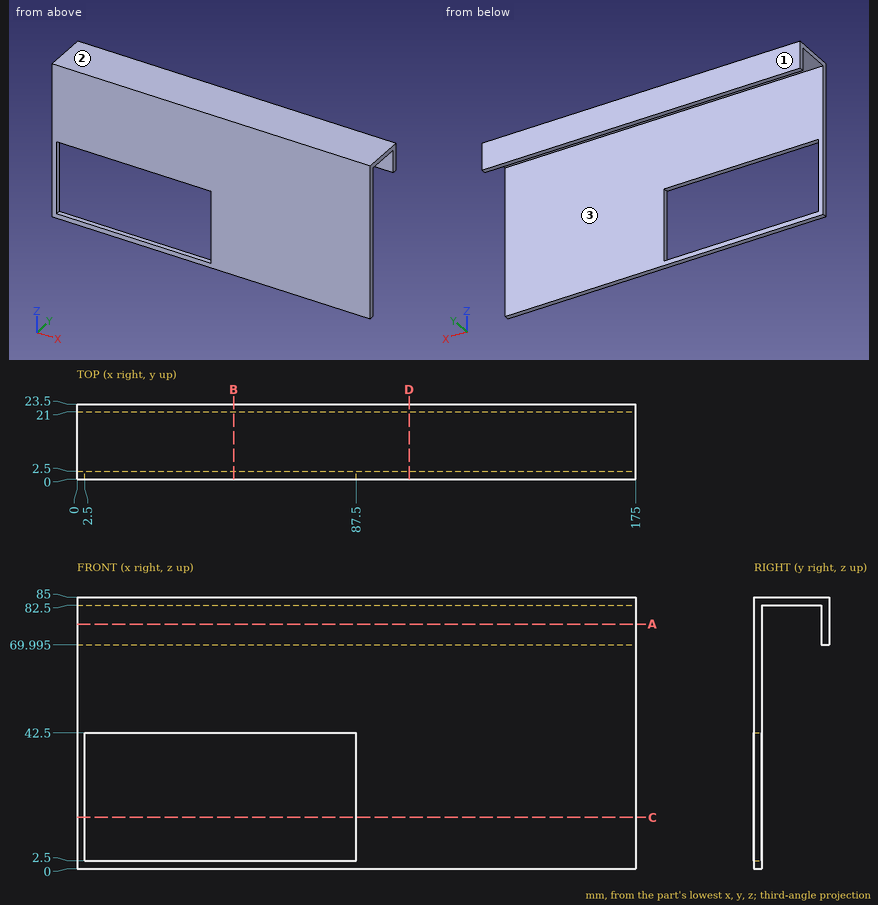
Geometry check sheet. Reference: drawing and pictorial views, mm from the part's lowest x, y, z. Give positions to 0.01 mm unless a question says otherwise; leave off trailing zeros. Order: outer loops, then holes, each group sorted by start corner. A loop starts at its lowest first (then second) coordinate and runs counter-clockwise, first axis right, second up. Notation, with made-up numbers: (-39, 65) -> (-11, 65) arc R19 cw to (-11, 78) -> close; hole circle Ø3 at (54, -33.5). An arc over 180 degrees is marked (long way). Use CSV: the item, a comma, the result in double quotes. Start each with the question number.
1) Go/stop test with flat-tipped pins: P1, Ø0.8, axis at y = 1, z = 19, coming from the -X side; P2, Ø6, axis at x = 48.5, z = 47.5, coming from the +Y side; P3, Ø3, axis at x = 61.5, y = 22, coming from the -Z side (3 decimals); P4, Ø12, axis at x = 61.5, y = 13.5, coming from the -Z side. Record where each tip stops, or that it passes through.
2) Sectioned sample at A-A, the plane z = 76.5. Record the boundary of the cut face in (x, y), plus the area to 3 significant figures.
3) Mould release check, pull along Y, two halves, no side actions. Record for the marked faces 1, 2 and 3: released by +Y, released by -Y, zero draft, split by the parting line, or undercut.
4) Material ranges on line 1 (Y direction, x = 21, z = 77.5); line 2 (Z direction, x = 113.5, y = 7.25); line 3 (Y direction, x = 155, z = 44), recorded low to high. Write a range as from..to.
5) Sectioned sample at B-B, the plane x = 49. Record the boundary of the cut face in (y, z) (3 decimals), plus the area to 3 significant figures.
6) Sectioned sample at D-D, the plane x = 104. Record the boundary of the cut face in (y, z) (3 decimals).
7) Sectioned sample at C-C, the plane z = 16. Record the boundary of the cut face in (x, y).
Recorded:
1,P1,"x = 0"
1,P2,"y = 2.5"
1,P3,"z = 69.995"
1,P4,"z = 82.5"
2,outline,"(0, 0) -> (175, 0) -> (175, 2.5) -> (0, 2.5) -> close; (0, 21) -> (175, 21) -> (175, 23.5) -> (0, 23.5) -> close"
2,area,"875 mm2"
3,face 1,"released by +Y"
3,face 2,"zero draft"
3,face 3,"undercut"
4,line 1,"0..2.5, 21..23.5"
4,line 2,"82.5..85"
4,line 3,"0..2.5"
5,outline,"(0, 0) -> (2.5, 0) -> (2.5, 2.5) -> (0, 2.5) -> close; (0, 42.5) -> (2.5, 42.5) -> (2.5, 82.5) -> (21, 82.5) -> (21, 69.995) -> (23.5, 69.995) -> (23.5, 85) -> (0, 85) -> close"
5,area,"196 mm2"
6,outline,"(0, 0) -> (2.5, 0) -> (2.5, 82.5) -> (21, 82.5) -> (21, 69.995) -> (23.5, 69.995) -> (23.5, 85) -> (0, 85) -> close"
7,outline,"(0, 0) -> (2.5, 0) -> (2.5, 2.5) -> (0, 2.5) -> close; (87.5, 0) -> (175, 0) -> (175, 2.5) -> (87.5, 2.5) -> close"
